The model under review builds one solid part; all positions refer to its coordinate system, in mm. Face numbers are marked on the shaded views. A direction names the side the tool comes from. Give positions to 0.01 mm unless a question says otherwise; leave off trailing zeros. Order: outer loops, then holes, each group sorted by start corner. A loop starts at its lowest first (then second) coordinate and runs counter-clockwise, first axis right, second up. Notation, with made-up numbers: (35.25, 38) - (78.25, 38) arc R25 ccw to (78.25, 74) - close; hole circle Ø8 at (48, -17.5). An arc over 180 degrees is marked (long way). Write item = value, one per line. Start each with the question number.
1. We need section A-A, the plane x = 92.5. Give the boundary of the cut face in (y, z), and give its area (3 significant figures).
2. We need section B-B, the plane z = 81. Give the boundary of the cut face in (x, y).
3. Machinability: for the marked faces 4, 5 and 6, which of the approach directions +Z, -Z, +X, -X, +Y, -Y give a long, thin tool a straight path to every point of the face, cutting with its end or side? Answer none if there is none.
4. We need section D-D, the plane x = -17.5. Give the boundary of the cut face in (y, z), and give its area (3 significant figures).
5. For P1, Ø22.5, axis at x = -19.5, y = 12.5, coming from the +Z side; P2, Ø8, axis at x = 80.5, y = -25.5, coming from the -Z side; P3, Ø5, axis at x = 8.5, y = -48.5, coming from the +Z side; P4, Ø6, axis at x = 77, z = 210, coming from the +Y side, all flat-tipped, find the tip position at first contact; note any pin that passes through.
6. Mouldability with a two-part tool opening along Z and no side actions: class the marked faces 1, 2 and 3 as pulls with the +Z half, pulls with the -Z half, needs draft (parallel to the pull), parting line crosses it, or undercut.
7. We need section C-C, the plane y = 0. Give the boundary of the cut face in (x, z), and give its area (3 significant figures).
8. Wall thickness on probe 1 along X at (y, z) = (-55, 292); probe 2 along X at (y, z) = (-50, 190.5); probe 3 along Y at (x, z) = (6, 27): over which ranges is each line inside the solid? List them lowest first.
from build123d import *

# Parameters (mm, degrees)
SKETCH2_R           = 44.45
BOSS_EXTRUDE1_DEPTH = 13.462
BOSS_EXTRUDE2_DEPTH = 38.1
SKETCH4_W           = 38.1
SKETCH4_H           = 66.04
BOSS_EXTRUDE3_DEPTH = 141.859
SKETCH5_W           = 66.04
SKETCH5_H           = 66.04
BOSS_EXTRUDE4_DEPTH = 43.6626
FILLET1_R           = 25.4
FILLET2_R           = 12.7
FILLET4_R           = 38.1
BOSS_EXTRUDE5_DEPTH = 66.04
SKETCH12_R          = 46.99
BOSS_EXTRUDE6_DEPTH = 5.969


with BuildPart() as part:
    # Sketch2 → Boss-Extrude1 (new body)
    with BuildSketch(Plane.XY):
        Circle(SKETCH2_R)
    extrude(amount=BOSS_EXTRUDE1_DEPTH)

    # Sketch3 → Boss-Extrude2 (add)
    with BuildSketch(Plane.XY.offset(13.462)):
        with BuildLine():
            Line((0, 33.02), (0, -33.02))
            ThreePointArc((0, -33.02), (-33.02, 0), (0, 33.02))
        make_face()
    extrude(amount=BOSS_EXTRUDE2_DEPTH)

    # Sketch4 → Boss-Extrude3 (add)
    with BuildSketch(Plane(origin=(0, 0, 0), x_dir=(0, 0, -1), z_dir=(1, 0, 0))):
        with Locations((-32.512, 0)):
            Rectangle(SKETCH4_W, SKETCH4_H)
    extrude(amount=BOSS_EXTRUDE3_DEPTH)

    # Sketch5 → Boss-Extrude4 (add)
    with BuildSketch(Plane(origin=(0, 18.542, 51.562), x_dir=(1, 0, 0), z_dir=(0, 0, -1))):
        with Locations((108.839, 18.542)):
            Rectangle(SKETCH5_W, SKETCH5_H)
    extrude(amount=-BOSS_EXTRUDE4_DEPTH)

    # Fillet1
    fillet1_edges = [part.edges().sort_by_distance(p)[0] for p in [
        (141.859, 0, 13.462),
    ]]
    fillet(fillet1_edges, radius=FILLET1_R)

    # Fillet2
    fillet2_edges = [part.edges().sort_by_distance(p)[0] for p in [
        (75.819, 0, 51.562),
    ]]
    fillet(fillet2_edges, radius=FILLET2_R)

    # Sketch8 → Loft1 section 0
    with BuildSketch(Plane(origin=(0, 0, 95.2246), x_dir=(0, -1, 0), z_dir=(0, 0, 1))):
        with BuildLine():
            Line((-33.02, 75.819), (33.02, 75.819))
            Line((33.02, 75.819), (33.02, 141.859))
            Line((33.02, 141.859), (-33.02, 141.859))
            Line((-33.02, 141.859), (-33.02, 75.819))
        make_face()
    # Sketch10 → Loft1 section 1
    with BuildSketch(Plane(origin=(0, -87.20411689, 293.962783253), x_dir=(-1, 0, 0), z_dir=(0, -0.2844002167201493, 0.958705646551397))):
        with BuildLine():
            Line((-141.859, 16.349067741), (-75.819, 16.349067741))
            Line((-75.819, 16.349067741), (-75.819, -49.690932259))
            Line((-75.819, -49.690932259), (-141.859, -49.690932259))
            Line((-141.859, -49.690932259), (-141.859, 16.349067741))
        make_face()
    loft()

    # Fillet4
    fillet4_edges = [part.edges().sort_by_distance(p)[0] for p in [
        (108.839, 33.02, 95.2246),
        (108.839, -33.02, 95.2246),
    ]]
    fillet(fillet4_edges, radius=FILLET4_R)

    # Sketch11 → Boss-Extrude5 (add)
    with BuildSketch(Plane(origin=(141.859, 0, 0), x_dir=(0, 0, -1), z_dir=(1, 0, 0))):
        with BuildLine():
            Line((-308.094895156, -39.565139551), (-289.313104844, -102.878060449))
            ThreePointArc((-289.313104844, -102.878060449), (-330.360460449, -80.612495156), (-308.094895156, -39.565139551))
        make_face()
    extrude(amount=-BOSS_EXTRUDE5_DEPTH)

    # Sketch12 → Boss-Extrude6 (add)
    with BuildSketch(Plane.ZY.offset(-75.819)):
        with Locations(Location((298.704, -71.2216, 0), (0, 0, 204.756785729))):
            Circle(SKETCH12_R)
    extrude(amount=BOSS_EXTRUDE6_DEPTH)


solid = part.part
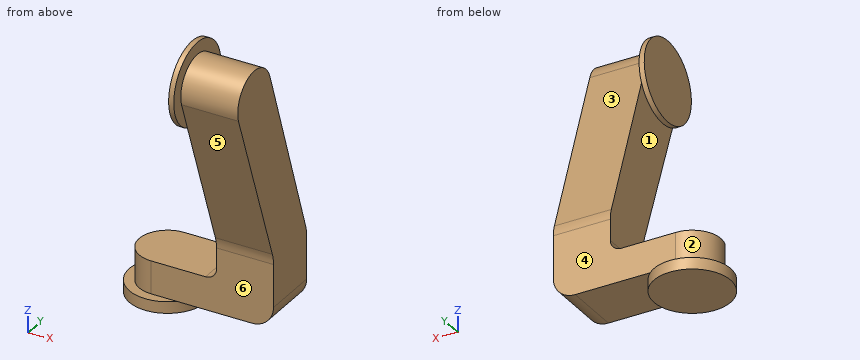
Model answer:
q1.outline = (-102.88, 289.31) - (-35.27, 101.48) arc R38.1 cw to (-33.02, 88.58) - (-33.02, 13.46) - (33.02, 13.46) - (33.02, 88.91) arc R38.1 ccw to (30.98, 101.2) - (-39.57, 308.09) arc R33.02 ccw to start
q1.area = 20,900 mm2
q2.outline = (75.82, -33.02) - (141.86, -33.02) - (141.86, 33.02) - (75.82, 33.02) - close
q3.face_4 = +Z, +X, -X, +Y
q3.face_5 = -Z, +X, -Y
q3.face_6 = +X, -X, -Y
q4.outline = (-40.86, 0) - (40.86, 0) - (40.86, 13.46) - (28, 13.46) - (28, 51.56) - (-28, 51.56) - (-28, 13.46) - (-40.86, 13.46) - close
q4.area = 3,230 mm2
q5.P1 = 51.56
q5.P2 = 13.46
q5.P3 = through
q5.P4 = -5.09
q6.face_1 = undercut
q6.face_2 = needs draft
q6.face_3 = pulls with the +Z half
q7.outline = (-44.45, 0) - (44.45, 0) - (44.45, 13.46) - (116.46, 13.46) arc R25.4 ccw to (141.86, 38.86) - (141.86, 192.06) - (75.82, 192.06) - (75.82, 64.26) arc R12.7 cw to (63.12, 51.56) - (-33.02, 51.56) - (-33.02, 13.46) - (-44.45, 13.46) - close
q7.area = 17,000 mm2
q8.probe_1 = 69.85 to 141.86
q8.probe_2 = 75.82 to 141.86
q8.probe_3 = -33.02 to 33.02
